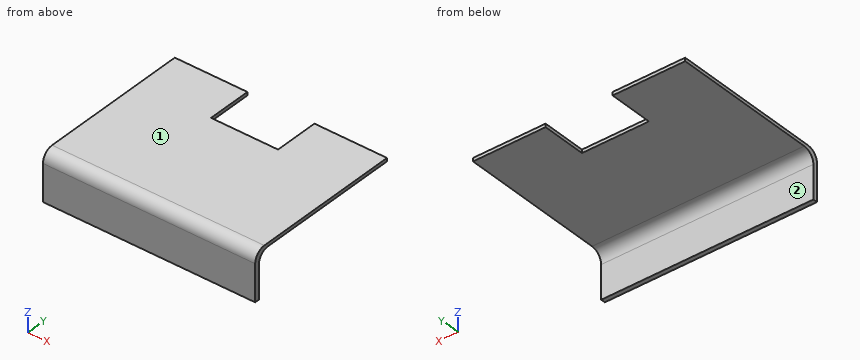
Autodesk Inventor part; units mm, degrees
ref_plane "YZ Plane" through (0, 0, 0) normal (1, 0, 0) x (0, 1, 0)
ref_plane "XZ Plane" through (0, 0, 0) normal (0, 1, 0) x (-1, 0, 0)
ref_plane "XY Plane" through (0, 0, 0) normal (0, 0, 1) x (1, 0, 0)
sketch "Sketch1" plane through (0, 0, 0) normal (0, 0, 1) x (1, 0, 0)
  line L0 (-15.6474, 9.6574) -> (174.3526, 9.6574)
  line L1 (174.3526, 9.6574) -> (174.3526, -135.3426)
  line L2 (174.3526, -135.3426) -> (-15.6474, -135.3426)
  line L3 (-15.6474, -135.3426) -> (-15.6474, 9.6574)
  line L4 (49.3526, 9.6574) -> (109.3526, 9.6574)
  line L5 (109.3526, 9.6574) -> (109.3526, -30.3426)
  line L6 (109.3526, -30.3426) -> (49.3526, -30.3426)
  line L7 (49.3526, -30.3426) -> (49.3526, 9.6574)
  point P0 (0, 0)
  dimension "d0" = 190
  dimension "d1" = 145
  dimension "d2" = 60
  dimension "d3" = 40
  dimension "d4" = 65
extrude "Extrusion1" add sketch "Sketch1" along normal blind 3 contours L0 L7 L6 L5 L1 L2 L3
sketch "Sketch2" plane through (0, 0, 0) normal (0, 0, -1) x (-1, 0, 0)
  line L0 (15.6474, -135.3426) -> (-174.3526, -135.3426)
  line L1 (-174.3526, -135.3426) -> (-174.3526, 9.6574)
  line L2 (15.6474, -135.3426) -> (-174.3526, -135.3426)
  line L3 (-174.3526, -135.3426) -> (-174.3526, -131.3426)
  line L4 (-174.3526, -131.3426) -> (15.6474, -131.3426)
  line L5 (15.6474, -131.3426) -> (15.6474, -135.3426)
  point P0 (0, 0)
  dimension "d7" = 4
extrude "Extrusion2" add sketch "Sketch2" along normal blind 40
fillet "Fillet1" radius 10 2 edges at (79.3526, -131.3426, 0) (79.3526, -135.3426, 3)
properties part number "płyta_dla_arduino"
Model file for the job. Use its own axes, mm. Face numbers are marked on the shaded views. A direction names the side the tool comes from. Give positions to 0.01 mm unless a question says otherwise; leave off trailing zeros. Order: outer loops, then holes, each group sorted by start corner. A loop starts at its lowest first (then second) coordinate and runs counter-clockwise, first axis right, second up.
1) Saw through at D-D, the plane x = 68.5. Write the cut outline in (y, z).
2) Saw through at B-B, the plane x = 129.5. Write the cut outline in (y, z), then the cut area to 3 significant figures.
3) Saw through at A-A, the plane y = -22.5. Write the cut outline in (x, z), then the cut area to 3 significant figures.
4) Pin check, flat tips, straight feed: pin 1 (8 mm diameter, centred on x = 146, y = -32, fed in from -Z); pin 2 (6 mm diameter, centred on x = 105.5, z = -17, fed in from +Y); pin 3 (2.5 mm diameter, centred on x = 72, z = 1.5, fed in from +Y). Stop position of each tip, or through.
5) Saw through at C-C, the plane z = -27. Write the cut outline in (x, y), then the cut area to 3 significant figures.
6) 3-axis set-ups, long thin cutter, end or side, ignore diameter. For the marked faces 1 and 2: which of +Z, -Z, +X, -X, +Y, -Y reach the whole face in a straight line?
7) Wall check: probe 1 along Y at (x, z) = (65, -14); probe 2 along Z at (x, y) = (15, -10.5); probe 3 along Z at (x, y) = (154.5, -124). Give the ranges that are in metal, low to high.
Computed:
1. outline: (-135.34, -40) - (-131.34, -40) - (-131.34, -10) arc R10 cw to (-121.34, 0) - (-30.34, 0) - (-30.34, 3) - (-125.34, 3) arc R10 ccw to (-135.34, -7) - close
2. outline: (-135.34, -40) - (-131.34, -40) - (-131.34, -10) arc R10 cw to (-121.34, 0) - (9.66, 0) - (9.66, 3) - (-125.34, 3) arc R10 ccw to (-135.34, -7) - close
2. area: 595 mm2
3. outline: (-15.65, 0) - (49.35, 0) - (49.35, 3) - (-15.65, 3) - close; (109.35, 0) - (174.35, 0) - (174.35, 3) - (109.35, 3) - close
3. area: 390 mm2
4. pin 1: stops at z = 0
4. pin 2: stops at y = -131.34
4. pin 3: stops at y = -30.34
5. outline: (-15.65, -135.34) - (174.35, -135.34) - (174.35, -131.34) - (-15.65, -131.34) - close
5. area: 760 mm2
6. face 1: +Z, +X, -X, +Y, -Y
6. face 2: -Z, +X, -X, +Y
7. probe 1: y = -135.34 to -131.34
7. probe 2: z = 0 to 3
7. probe 3: z = -0.36 to 3
